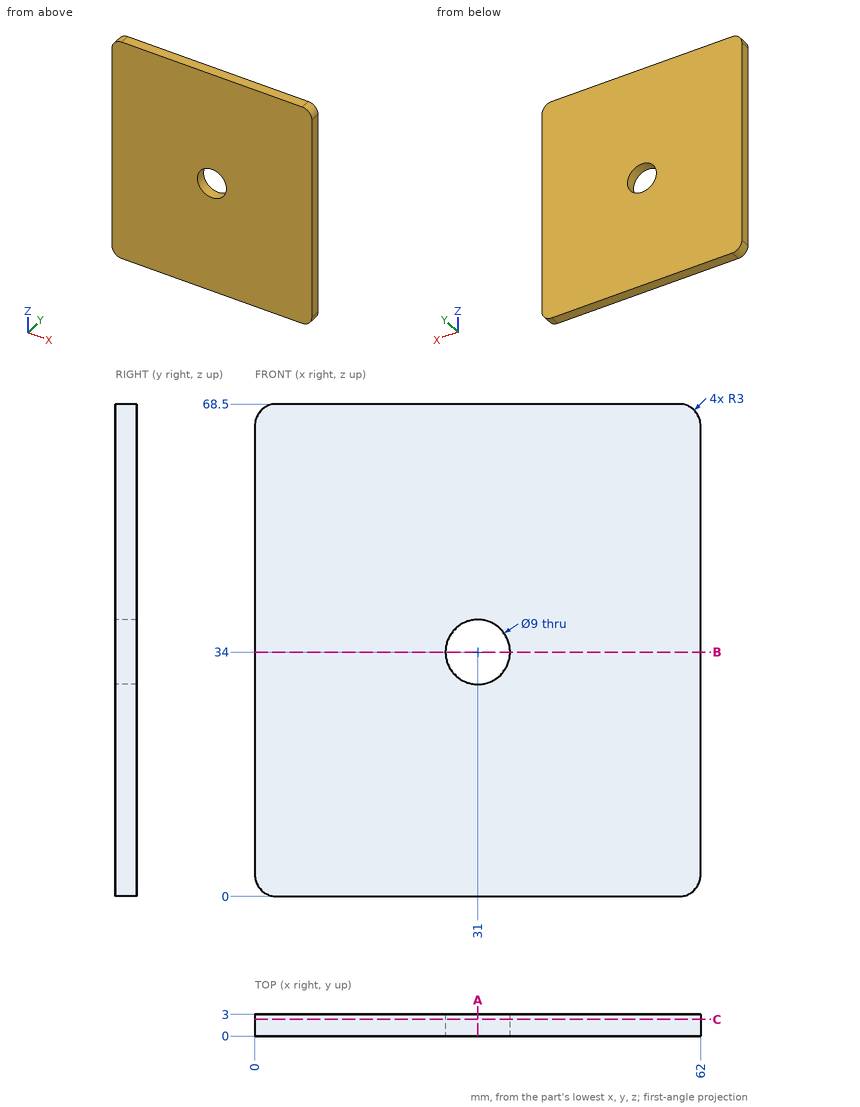
The figure shows three views and two pictorial views of one solid part (mm, origin at its lowest corner). Answer the questions. Coordinates: 2 decimals unless noted, no trailing zeros. Write each loop counter-clockwise with the first axis right and the second up, starting at its lowest first coordinate (ties: lowest second). Pieces come first, ordered by that corner, then holes. Notation, with made-up numbers: (23, 66.5) -> (30, 66.5) arc R19 ccw to (30, 103.5) -> close; hole circle Ø3 at (-16, -39). An arc over 180 degrees is marked (long way). Return JSON: item names as keys, results as strings.
(1) The part is cut by section A-A on x = 31. Give the vertices of the cut face in (y, z).
Answers below:
{"outline": "(0, 0) -> (3, 0) -> (3, 29.5) -> (0, 29.5) -> close; (0, 38.5) -> (3, 38.5) -> (3, 68.5) -> (0, 68.5) -> close"}
(2) The part is cut by section C-C on y = 2.3. Give the vertices of the cut face in (x, z).
Answers below:
{"outline": "(0, 3) arc R3 ccw to (3, 0) -> (59, 0) arc R3 ccw to (62, 3) -> (62, 65.5) arc R3 ccw to (59, 68.5) -> (3, 68.5) arc R3 ccw to (0, 65.5) -> close; hole circle Ø9 at (31, 34)"}
(3) Consider line 1 along Z through (x, y) = (31, 2). Determine where the line is inside the solid, lowest interval first. Write a range as from..to.
Answers below:
{"line 1": "0..29.5, 38.5..68.5"}
(4) The part is cut by section B-B on z = 34. Give the vertices of the cut face in (x, y), then the cut area to 3 significant figures.
Answers below:
{"outline": "(0, 0) -> (26.5, 0) -> (26.5, 3) -> (0, 3) -> close; (35.5, 0) -> (62, 0) -> (62, 3) -> (35.5, 3) -> close", "area": "159 mm^2"}
